```python
from build123d import *

# Parameters (mm, degrees)
F1_DEPTH = 5.08


with BuildPart() as f1:
    # F0 (on Front) → F1 (new body)
    with BuildSketch(Plane.XZ):
        with BuildLine():
            Line((0, 12.728863), (0, 12.714432))
            ThreePointArc((0, 12.714432), (-1.859872, 8.224304), (-6.35, 6.364432))
            Line((-6.35, 6.364432), (-22.579235, 6.364432))
            ThreePointArc((-22.579235, 6.364432), (-27.069363, 4.50456), (-28.929235, 0.014432))
            Line((-28.929235, 0.014432), (-28.929235, 0))
            Line((-28.929235, 0), (0, 0))
            Line((0, 0), (57.858475, 0))
            Line((57.858475, 0), (57.858475, 6.378863))
            ThreePointArc((57.858475, 6.378863), (55.998604, 10.868991), (51.508475, 12.728863))
            Line((51.508475, 12.728863), (45.129612, 12.728863))
            Line((45.129612, 12.728863), (0, 12.728863))
        make_face()
        with BuildLine():
            Line((0, 0), (-28.929235, 0))
            Line((-28.929235, 0), (-28.929235, -0.014432))
            ThreePointArc((-28.929235, -0.014432), (-27.069363, -4.50456), (-22.579235, -6.364432))
            Line((-22.579235, -6.364432), (-6.35, -6.364432))
            ThreePointArc((-6.35, -6.364432), (-1.859872, -8.224304), (0, -12.714432))
            Line((0, -12.714432), (0, -12.728863))
            Line((0, -12.728863), (45.129612, -12.728863))
            Line((45.129612, -12.728863), (51.508475, -12.728863))
            ThreePointArc((51.508475, -12.728863), (55.998604, -10.868991), (57.858475, -6.378863))
            Line((57.858475, -6.378863), (57.858475, 0))
            Line((57.858475, 0), (0, 0))
        make_face()
    extrude(amount=F1_DEPTH)


solid = f1.part
```
Input: part model. Units: mm. Frame: model coordinates. A direction names the side the tool comes from. Give positions to 0.01 mm unless a question says otherwise; leave off trailing zeros. Write each loop counter-clockwise with the first axis right and the second up, starting at its lowest first coordinate (ties: lowest second). Pieces come first, ordered by that corner, then holes. Notation, with made-up numbers: (-14, 18.5) - (-1, 18.5) arc R15 cw to (-1, 25.5) - close; hole circle Ø11 at (-26, 27). An arc over 180 degrees is marked (long way). Write item = value, one per line. Start each with the question number.
1. Section query C-C, the plane z = -9. Output: boundary loops of the cut face in (x, y).
2. First-contact query: pin 1 Ø3 at (y, z) = (-3.5, 5) entering from -X; pin 2 Ø1.5 at (x, y) = (-16.5, -3.5) entering from +Z; pin 3 Ø6 at (x, z) = (9, -6) entering from +Y. Flat tips, straight axial feed; report the tip coordinate or a pass-through.
3. Mould query, pull axis Z, two halves, no side actions, for faces 3 (the cylindrical face through (-27.118, -2.504, -4.455)), 4 (the flat face through (24, 0, 0)), 5 (the flat face through (-14, -3, 6.364)). Classes: released by +Z, released by -Z, zero draft, split by the parting line, or undercut.
4. Ray query, L1, parallel to Z at x = -22, y = -1.7; L2, parallel to X at y = -0.75, z = -8; L3, parallel to X at y = -1.35, z = -7.5. Return the intervals inside material, ascending.
5. Section query B-B, the plane x = -14. Output: boundary loops of the cut face in (y, z).
6. Access query for faces 1 (the flat face through (-15, -3, -6.364)), 2 (the flat face through (57.858, -3, 0)). Directions: +Z, -Z, +X, -X, +Y, -Y. A direction counts if a zero-diameter tool reaches every point of the face in a straight line with its end or side. Return the directions, or none.
Check sheet entries:
q1.outline = (-1.2, -5.08) - (57.29, -5.08) - (57.29, 0) - (-1.2, 0) - close
q2.pin_1 = -27.89
q2.pin_2 = 6.36
q2.pin_3 = 0
q3.face_3 = released by -Z
q3.face_4 = zero draft
q3.face_5 = released by +Z
q4.L1 = -6.36 to 6.36
q4.L2 = -2.1 to 57.65
q4.L3 = -2.73 to 57.76
q5.outline = (-5.08, -6.36) - (0, -6.36) - (0, 6.36) - (-5.08, 6.36) - close
q6.face_1 = -Z, -X, +Y, -Y
q6.face_2 = +Z, -Z, +X, +Y, -Y
